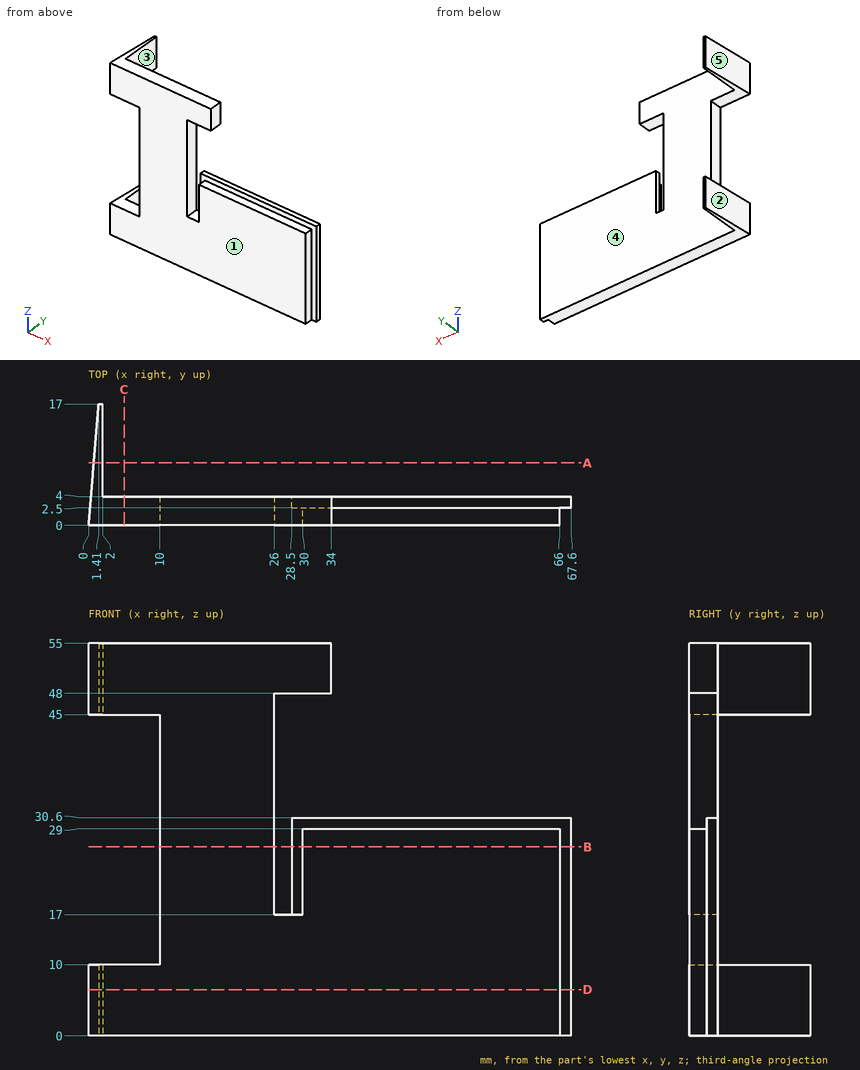
The figure shows three views and two pictorial views of one solid part (mm, origin at its lowest corner). Answer the questions. A direction names the side the tool comes from. Coordinates: 2 decimals unless noted, no trailing zeros. Write each loop counter-clockwise with the first axis right and the second up, starting at its lowest first coordinate (ties: lowest second). Pieces come first, ordered by that corner, then holes. Notation, with made-up numbers: (22, 70) -> (58, 70) arc R26 cw to (58, 101) -> close; hole circle Ø5 at (31.5, 60). An arc over 180 degrees is marked (long way). Return JSON: item names as keys, results as strings.
1. A tool of negligible diameter and unlimited length cuts with its end or side. For the marked faces 4 and 5, from which of +Z, -Z, +X, -X, +Y, -Y can it reach the whole face along a straight path? Write none if from no direction.
Found:
{"face 4": "+Z, -Z, +X, +Y", "face 5": "+Z, -Z, -X, +Y"}
2. A cutting plane is placed at B-B (z = 26.5). Determine the outline of the cut face in (x, y).
Found:
{"outline": "(10, 0) -> (26, 0) -> (26, 4) -> (10, 4) -> close; (28.5, 2.5) -> (30, 2.5) -> (30, 0) -> (66, 0) -> (66, 2.5) -> (67.6, 2.5) -> (67.6, 4) -> (28.5, 4) -> close"}
3. A cutting plane is placed at A-A (y = 8.75). Determine the outline of the cut face in (x, z), and give its area (3 significant figures).
Found:
{"outline": "(0.73, 0) -> (2, 0) -> (2, 10) -> (0.73, 10) -> close; (0.73, 45) -> (2, 45) -> (2, 55) -> (0.73, 55) -> close", "area": "25.5 mm2"}
4. Each of these flat-tipped pins is pushed along its axis until it touches: P1, Ø1.2, axis at y = 2, z = 50, coming from the +X side; P2, Ø0.8, axis at x = 50.5, y = 2, coming from the +Z side; P3, Ø2, axis at y = 3, z = 29.5, coming from the -X side. Where does it stop, or does it pass through?
Found:
{"P1": "x = 34", "P2": "z = 29", "P3": "x = 10"}
5. Determine the mould class of the marked faces 1, 2 and 3 for opening direction X: pulls with the +X half, pulls with the -X half, needs draft (parallel to the pull), parting line crosses it, or undercut.
Found:
{"face 1": "needs draft", "face 2": "pulls with the -X half", "face 3": "pulls with the +X half"}
6. A cutting plane is placed at D-D (z = 6.5). Determine the outline of the cut face in (x, y), and give its area (3 significant figures).
Found:
{"outline": "(0, 0) -> (66, 0) -> (66, 2.5) -> (67.6, 2.5) -> (67.6, 4) -> (2, 4) -> (2, 17) -> (1.41, 17) -> close", "area": "280 mm2"}
7. Find the intervals of material crossed by line 1 along Y through (x, z) = (12, 38); line 2 along X through (y, z) = (1.75, 38); line 3 along X through (y, z) = (8.25, 51), in increasing order. Write a range as from..to.
Found:
{"line 1": "0..4", "line 2": "10..26", "line 3": "0.68..2"}
8. A cutting plane is placed at C-C (x = 5). Determine the outline of the cut face in (y, z), and give its area (3 significant figures).
Found:
{"outline": "(0, 0) -> (4, 0) -> (4, 10) -> (0, 10) -> close; (0, 45) -> (4, 45) -> (4, 55) -> (0, 55) -> close", "area": "80.0 mm2"}
